Verification items for this drawing (mm, ordinates from the low corner). Give positions to 0.01 mm unless a question says otherwise; leave off trailing zeros. Order: outer loops, then holes, each group sorted by start corner. A loop starts at its lowest first (then second) coordinate and runs counter-clockwise, first axis right, second up. Notation, with made-up numbers: M 48,-36 L 102,-36 A31 cw 102,-2 Z; hole C -11.5,-1 d7. An arc over 180 degrees is marked long. Answer as a JSON object with one key per item and string values.
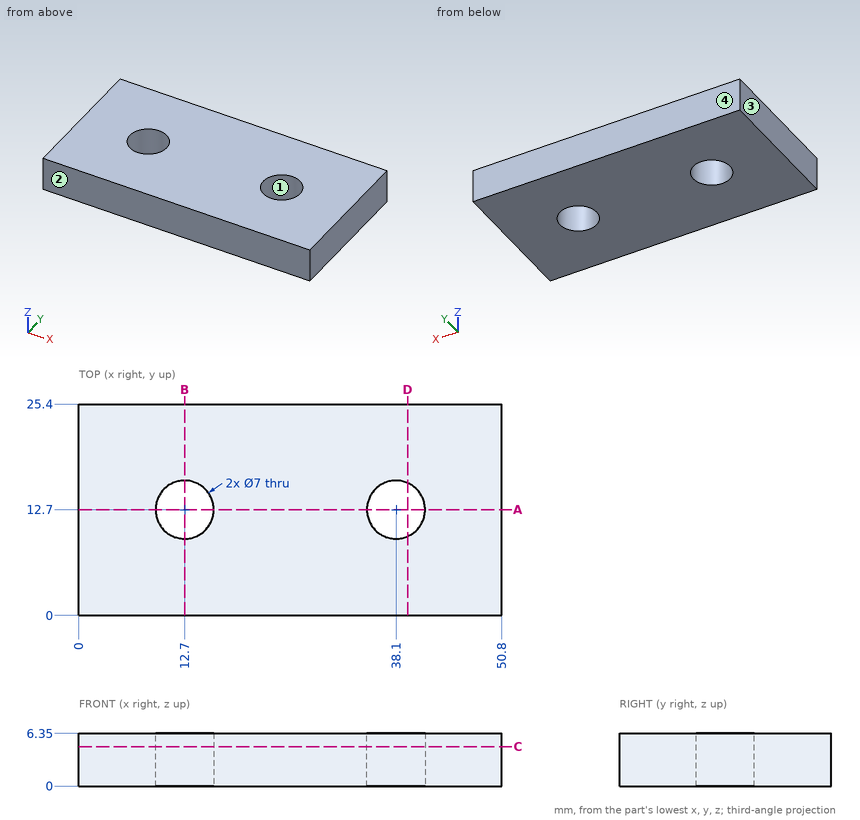
Q1. Section check B-B on x = 12.7. Record the cut outline in (y, z).
Resolved:
{"outline": "M 0,0 L 9.2,0 L 9.2,6.35 L 0,6.35 Z; M 16.2,0 L 25.4,0 L 25.4,6.35 L 16.2,6.35 Z"}
Q2. Gauge pin test, flat end, axial feed: pin 1 Ø1.5 at (x, y) = (38.5, 12) entering from -Z. Record the tip position at first contact, or that the pin passes through.
Resolved:
{"pin 1": "passes through"}
Q3. Section check C-C on z = 4.75. Record the cut outline in (x, y), then the cut area to 3 significant figures.
Resolved:
{"outline": "M 0,0 L 50.8,0 L 50.8,25.4 L 0,25.4 Z; hole C 12.7,12.7 d7; hole C 38.1,12.7 d7", "area": "1,210 mm²"}
Q4. Section check D-D on x = 39.5. Record the cut outline in (y, z), then the cut area to 3 significant figures.
Resolved:
{"outline": "M 0,0 L 9.49,0 L 9.49,6.35 L 0,6.35 Z; M 15.91,0 L 25.4,0 L 25.4,6.35 L 15.91,6.35 Z", "area": "121 mm²"}
Q5. Release check for a two-part mould opening along Y. For the marked faces 1, 2, 3 and 4 record: +Y half, -Y half, draft (parallel to the pull), parting line (faces both ways), or undercut.
Resolved:
{"face 1": "undercut", "face 2": "-Y half", "face 3": "draft", "face 4": "+Y half"}
Q6. Section check A-A on y = 12.7. Record the cut outline in (x, z).
Resolved:
{"outline": "M 0,0 L 9.2,0 L 9.2,6.35 L 0,6.35 Z; M 16.2,0 L 34.6,0 L 34.6,6.35 L 16.2,6.35 Z; M 41.6,0 L 50.8,0 L 50.8,6.35 L 41.6,6.35 Z"}
Q7. Material ranges on L1, parallel to X at y = 11.75, z = 2.25; L2, parallel to Y at x = 38.1, z = 4.75; L3, parallel to Y at x = 11, z = 2.5, recorded low to high.
Resolved:
{"L1": "x = 0 to 9.33, 16.07 to 34.73, 41.47 to 50.8", "L2": "y = 0 to 9.2, 16.2 to 25.4", "L3": "y = 0 to 9.64, 15.76 to 25.4"}
